```python
from build123d import *

# Parameters (mm, degrees)
SKETCH1_W           = 56
SKETCH1_H           = 15
BOSS_EXTRUDE1_DEPTH = 14
SKETCH2_R           = 4.375
CUT_EXTRUDE1_DEPTH  = 28
SKETCH4_R           = 3
CUT_EXTRUDE3_DEPTH  = 15
CUT_EXTRUDE4_DEPTH  = 3.375


with BuildPart() as part:
    # Sketch1 → Boss-Extrude1 (new, symmetric)
    with BuildSketch(Plane(origin=(0, 0, 0), x_dir=(1, 0, 0), z_dir=(0, 1, 0))):
        Polygon((-16.35, 15.7), (-12.171891314, 7.5), (12.171891314, 7.5), (16.35, 15.7), align=None)
        Rectangle(SKETCH1_W, SKETCH1_H)
    extrude(amount=BOSS_EXTRUDE1_DEPTH, both=True)

    # Sketch2 → Cut-Extrude1 (cut)
    with BuildSketch(Plane(origin=(0, 14, 0), x_dir=(1, 0, 0), z_dir=(0, 1, 0))):
        with Locations(Location((0, 5.7, 0), (0, 0, 270))):
            Circle(SKETCH2_R)
    extrude(amount=-CUT_EXTRUDE1_DEPTH, mode=Mode.SUBTRACT)

    # Sketch4 → Cut-Extrude3 (cut)
    with BuildSketch(Plane.XY.offset(7.5)):
        with Locations((-21, 0)):
            Circle(SKETCH4_R)
        with Locations((21, 0)):
            Circle(SKETCH4_R)
    extrude(amount=-CUT_EXTRUDE3_DEPTH, mode=Mode.SUBTRACT)

    # Sketch3 → Cut-Extrude4 (cut, symmetric)
    with BuildSketch(Plane.XZ):
        Polygon((7.505553499, -5.7), (7.505553499, -15.7), (-7.505553499, -15.7), (-7.505553499, -5.7), (-3.75277675, 0.8), (3.75277675, 0.8), align=None)
    extrude(amount=CUT_EXTRUDE4_DEPTH, both=True, mode=Mode.SUBTRACT)


solid = part.part
```
Build history of the part. All positions in model axes, mm. A direction names the side the tool comes from. Round coordinates to 2 decimals unless told otherwise and drop trailing zeros. Loops run counter-clockwise (first coordinate to the right, second up) from the corner with the lowest first, then second, coordinate; pieces in that order, holes last.
Item 1: Drill centre lines: line 1 along Y through (x, z) = (-21, -2.25); line 2 along X through (y, z) = (7.5, -5.7) (3 decimals); line 3 along X through (y, z) = (-2, 6). Where is each one in solid material? Low to high.
Item 2: Saw through at A-A (x = 21). List the corners of the cut face in (y, z), then the cut area to 3 significant figures.
Item 3: Saw through at B-B (z = -2.5). List the corners of the cut face in (x, y) (3 decimals).
Item 4: Which spindle directions (+Z, -Z, +X, -X, +Y, -Y) get a long thin tool onto all of the face, cutting with end or side? Do faces 4 (the face through (5.6, 0, -2.4)), 5 (the face through (14.23, 0.2, -11.54)), 6 (the face through (-14.29, 0.2, -11.66)), 7 (the face through (1.314, -8.613, -1.527)). Say none if no direction does.
Item 5: Pin check, flat tips, straight feed: P1, Ø3.5, axis at y = 1, z = -9.5, coming from the -X side; P2, Ø5.5, axis at y = 1.5, z = -10.5, coming from the +X side; P3, Ø4.5, axis at x = 22, y = -4.5, coming from the -Z side. Stop position of each tip, or through.
Item 6: Saw through at D-D (y = 4.5). List the corners of the cut face in (x, z) (3 decimals), then the cut area to 3 significant figures.
Item 7: Two-plate mould, pull along Z, no slides. Class faces 1 (the face through (0, 6, -15.7)), 2 (the face through (7.506, 0, -11)), 3 (the face through (-20, 3, -7.5)): released by +Z, released by -Z, zero draft, split by the parting line, or undercut.
Item 8: Saw through at C-C (x = 0). List the corners of the cut face in (y, z) (3 decimals), then the cut area to 3 significant figures.
Worked answers:
1. line 1: y = -14 to -3, 3 to 14
1. line 2: x = -28 to -4.375, 4.375 to 28
1. line 3: x = -28 to -23.24, -18.76 to 18.76, 23.24 to 28
2. outline: (-14, -7.5) - (-3, -7.5) - (-3, 7.5) - (-14, 7.5) - close; (3, -7.5) - (14, -7.5) - (14, 7.5) - (3, 7.5) - close
2. area: 330 mm2
3. outline: (-28, -14) - (-2.983, -14) - (-2.983, -3.375) - (-5.658, -3.375) - (-5.658, 3.375) - (-2.983, 3.375) - (-2.983, 14) - (-28, 14) - close; (2.983, -14) - (28, -14) - (28, 14) - (2.983, 14) - (2.983, 3.375) - (5.658, 3.375) - (5.658, -3.375) - (2.983, -3.375) - close; hole circle Ø6 at (-21, 0); hole circle Ø6 at (21, 0)
4. face 4: -Z
4. face 5: +X, +Y, -Y
4. face 6: -X, +Y, -Y
4. face 7: +Y, -Y
5. P1: stops at x = -14.08
5. P2: stops at x = 15.1
5. P3: stops at z = -7.5
6. outline: (-28, -7.5) - (-12.172, -7.5) - (-16.35, -15.7) - (16.35, -15.7) - (12.172, -7.5) - (28, -7.5) - (28, 7.5) - (-28, 7.5) - close; hole circle Ø8.75 at (0, -5.7)
6. area: 1,010 mm2
7. face 1: released by -Z
7. face 2: zero draft
7. face 3: undercut
8. outline: (-14, -15.7) - (-3.375, -15.7) - (-3.375, -10.075) - (-14, -10.075) - close; (-14, -1.325) - (-3.375, -1.325) - (-3.375, 0.8) - (3.375, 0.8) - (3.375, -1.325) - (14, -1.325) - (14, 7.5) - (-14, 7.5) - close; (3.375, -15.7) - (14, -15.7) - (14, -10.075) - (3.375, -10.075) - close
8. area: 352 mm2
